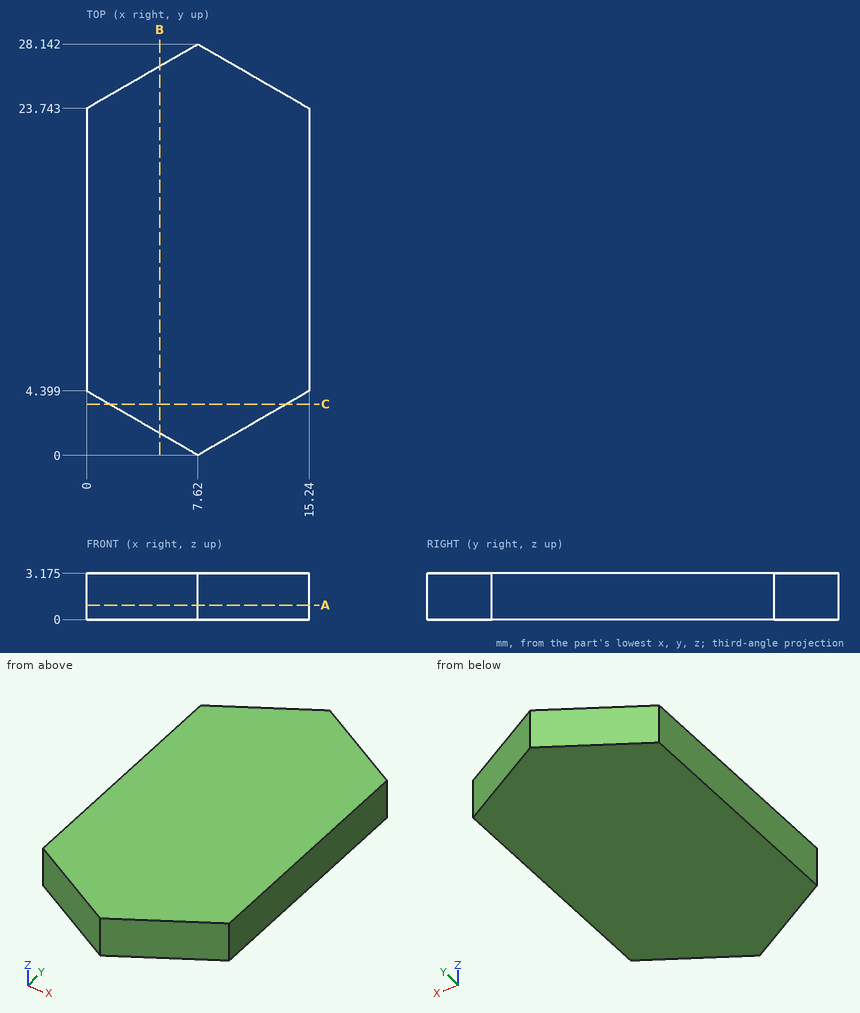
Part print with two shaded views. Sizes in mm from the minimum x, y, z corner. Give positions to 0.01 mm unless a question says otherwise; leave off trailing zeros. Order: outer loops, then holes, each group sorted by start corner. A loop starts at its lowest first (then second) coordinate and runs counter-clockwise, first axis right, second up.
(1) Drill centre lines: L1, parallel to Y at x = 4, z = 2; L2, parallel to X at y = 3, z = 1.6 (1 decimal); L3, parallel to Y at x = 5.75, z = 2.7 (1 decimal). Where is each one in solid material? Low to high.
(2) Saw through at A-A, the plane z = 1. Give the cut face in (x, y).
(3) Flat gauge pin, fed straight in: pin 1 (1 mm diameter, centred on x = 5.5, y = 10.5, fed in from -Z). Where does the tip first touch, or does it go through?
(4) Saw through at C-C, the plane y = 3.5. Give the cut face in (x, z) (1 decimal).
(5) Saw through at B-B, the plane x = 5. Give the cut face in (y, z) (1 decimal).
Results found:
1. L1: y = 2.09 to 26.05
1. L2: x = 2.4 to 12.8
1. L3: y = 1.1 to 27.1
2. outline: (0, 4.4) - (7.62, 0) - (15.24, 4.4) - (15.24, 23.74) - (7.62, 28.14) - (0, 23.74) - close
3. pin 1: stops at z = 0
4. outline: (1.6, 0) - (13.7, 0) - (13.7, 3.2) - (1.6, 3.2) - close
5. outline: (1.5, 0) - (26.6, 0) - (26.6, 3.2) - (1.5, 3.2) - close
